Design review of the part shown in the three views and the two pictorial views. Dimensions are in mm from the part's minimum x, y and z. Give positions to 0.01 mm unless a question says otherwise; leave off trailing zeros. Order: outer loops, then holes, each group sorted by start corner. A loop starts at its lowest first (then second) coordinate and runs counter-clockwise, first axis right, second up.
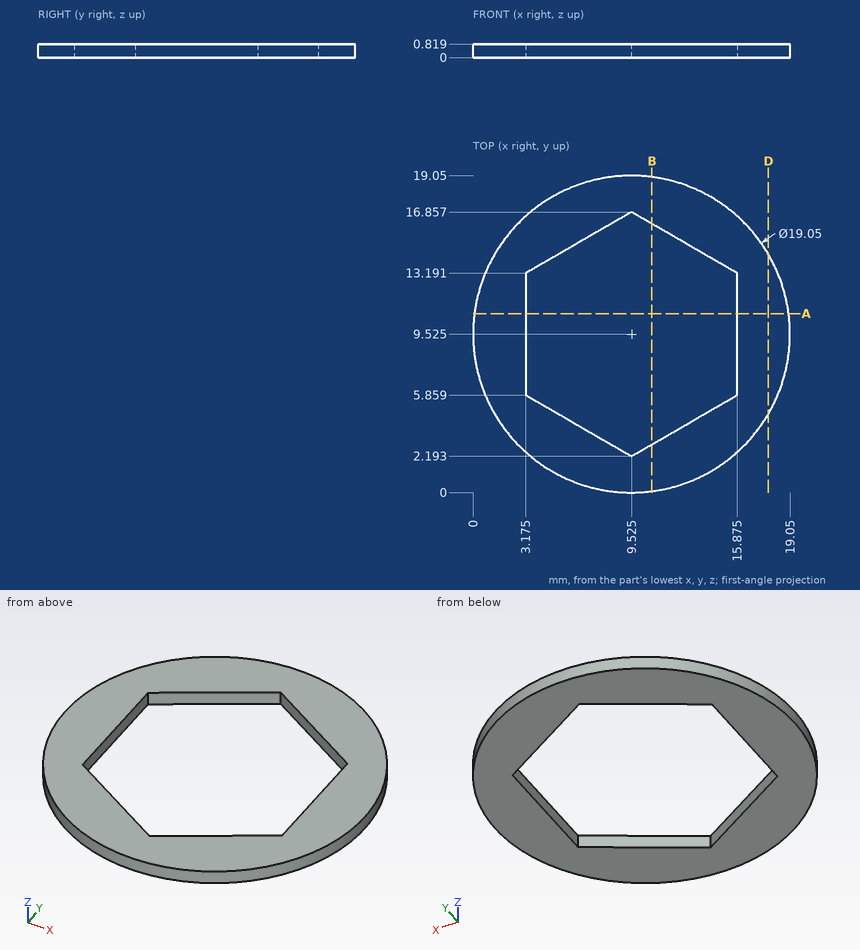
Item 1: For line 1 (Y direction, x = 14.75, z = 0.1); line 2 (Y direction, x = 6, z = 0.45) (1 decimal); line 3 (X direction, y = 6.25, z = 0.25) (1 decimal), list the stretches that pass through material, from the lowest coordinate up.
Values found:
line 1: y = 1.56 to 5.21, 13.84 to 17.49
line 2: y = 0.7 to 4.2, 14.8 to 18.4
line 3: x = 0.6 to 3.2, 15.9 to 18.5
Item 2: Take a section at A-A (y = 10.75). Give the boundary of the cut face in (x, z) (1 decimal).
Values found:
outline: (0.1, 0) - (3.2, 0) - (3.2, 0.8) - (0.1, 0.8) - close; (15.9, 0) - (19, 0) - (19, 0.8) - (15.9, 0.8) - close
Item 3: Take a section at D-D (x = 17.75). Give the boundary of the cut face in (y, z).
Values found:
outline: (4.72, 0) - (14.33, 0) - (14.33, 0.82) - (4.72, 0.82) - close
Item 4: Take a section at B-B (x = 10.75). Give the boundary of the cut face in (y, z).
Values found:
outline: (0.08, 0) - (2.9, 0) - (2.9, 0.82) - (0.08, 0.82) - close; (16.15, 0) - (18.97, 0) - (18.97, 0.82) - (16.15, 0.82) - close
